Autodesk Inventor part; units mm, degrees
ref_plane "to_bolt_XY" through (5, -9, 0) normal (1, 0, 0) x (0, 0, -1)
ref_plane "to_bolt_YZ" through (5, -9, 0) normal (0, 0, -1) x (0, 1, 0)
ref_plane "to_bolt_ZX" through (5, -9, 0) normal (0, 1, 0) x (1, 0, 0)
sketch "Sketch_14" plane through (0, 0, 0) normal (1, 0, 0) x (0, 1, 0)
  line L0 (0, -4) -> (0, 4)
  line L1 (0, 4) -> (14.5, 4)
  line L2 (14.5, 4) -> (15, 3.5)
  line L3 (15, 3.5) -> (15, -3.5)
  line L4 (15, -3.5) -> (14.5, -4)
  line L5 (14.5, -4) -> (0, -4)
  line L6 (0, -4) -> (0, 4)
revolve "Revolution1" add sketch "Sketch_14" angle 360 about axis through (0, 0, -4) along (0, 0, -1)
sketch "Sketch_15" plane through (0, 0, 0) normal (1, 0, 0) x (0, 1, 0)
  line L0 (0, -4) -> (0, 4)
  line L1 (0, 4) -> (5.5, 4)
  line L2 (5.5, 4) -> (5, 3.5)
  line L3 (5, 3.5) -> (5, -3.5)
  line L4 (5, -3.5) -> (5.5, -4)
  line L5 (5.5, -4) -> (0, -4)
  line L6 (0, -4) -> (0, 4)
revolve "Revolution2" cut sketch "Sketch_15" angle 360 about axis through (0, 0, -4) along (0, 0, -1)
sketch "Sketch_16" plane through (0, 0, 0) normal (0, 0, 1) x (1, 0, 0)
  arc A0 (-0.75, -15.9824) -> (0.75, -15.9824) centre (0, 0) ccw
  line L0 (0.75, -15.9824) -> (0.75, 0)
  line L1 (0.75, 0) -> (-0.75, 0)
  line L2 (-0.75, 0) -> (-0.75, -15.9824)
extrude "Extrusion1" cut sketch "Sketch_16" along normal mid plane 8
sketch "Sketch4" plane through (0, 0, -4) normal (0, 0, -1) x (-1, 0, 0)
  point P0 (-10, 0)
hole "Hole1" at (10, 0, -4) direction (0, 0, 1) diameter 5.5 depth 8
sketch "Sketch5" plane through (0, 0, -4) normal (0, 0, -1) x (-1, 0, 0)
  point P0 (10, 0)
hole "Hole2" at (-10, 0, -4) direction (0, 0, 1) diameter 5.5 depth 8
sketch "Sketch6" plane through (0, 0, -4) normal (0, 0, -1) x (-1, 0, 0)
  point P0 (0, 10)
hole "Hole3" at (0, 10, -4) direction (0, 0, 1) diameter 5.5 depth 8
sketch "Sketch_23" plane through (0, -9, 0) normal (0, 1, 0) x (1, 0, 0)
  line L0 (15, 0) -> (0, 0)
  line L1 (0, 0) -> (0, 1.7)
  line L2 (0, 1.7) -> (5, 1.7)
  line L3 (5, 1.7) -> (5, 3)
  line L4 (5, 3) -> (15, 3)
  line L5 (15, 3) -> (15, 0)
  line L6 (15, 0) -> (0, 0)
revolve "Revolution3" cut sketch "Sketch_23" angle 360 about axis through (15, -9, 0) along (1, 0, 0)
sketch "Sketch8" plane through (-0.75, -14.4806, 4) normal (1, 0, 0) x (0, 0, -1)
  point P0 (4, 5.4806)
hole "Hole4" at (-0.75, -9, 0) direction (-1, 0, 0) diameter 2.459 depth 12.2404 countersink diameter 3 countersink angle 90
ref_plane "to_bolt_XY" through (5, -9, 0) normal (1, 0, 0) x (0, 0, -1)
ref_plane "to_bolt_YZ" through (5, -9, 0) normal (0, 0, -1) x (0, 1, 0)
ref_plane "to_bolt_ZX" through (5, -9, 0) normal (0, 1, 0) x (1, 0, 0)
properties part number "SCST10-8b"
Verification items for the finished model (mm, model axes). A direction names the side the tool comes from. Coordinates: 2 decimals unless noted, no trailing zeros. Write each loop counter-clockwise with the first axis right and the second up, starting at its lowest first coordinate (ties: lowest second). Pieces come first, ordered by that corner, then holes. Notation, with made-up numbers: (57.5, 66) -> (97.5, 66) arc R30 cw to (97.5, 100) -> close; hole circle Ø1 at (74.5, 81). An arc over 180 degrees is marked (long way). One line per item, written item: value. Start each with the question number.
Q1. Thickness scan on L1, parallel to X at y = 0, z = -0.25; L2, parallel to Z at x = -7.25, y = -9; L3, parallel to Y at x = -1, z = 1.5. Record the ranges inside material, lowest first. Write a range as from..to.
Q2. Cross-section at A-A on y = 0. Enter the section's corners in (x, z).
Q3. Access from +Z, -Z, +X, -X, +Y, -Y to the whole of each face (thin tool, end or side, straight path). Record for faces 1 (the cylindrical face through (2.9, -10.66, 0.37)), 2 (the cylindrical face through (0, 5, 0)), 3 (the flat face through (0.75, -11, 0)).
Q4. Mould release check, pull along X, two halves, no side actions. Record for faces 4 (the flat face through (5, -11, 0)), 5 (the conical face through (-0.634, 14.629, 3.858)), 6 (the flat face through (-0.75, -11, 0)): pulls with the +X half, pulls with the -X half, needs draft (parallel to the pull), parting line crosses it, or undercut.
Q5. Go/stop test with flat-tipped pins: P1, Ø2, axis at y = -4, z = -2.5, coming from the +X side; P2, Ø1, axis at y = 7, z = 0, coming from the -X side; P3, Ø4.5, axis at y = -9, z = 0, coming from the +X side. Record where each tip stops, or that it passes through.
Q6. Cross-section at B-B on x = -3.5. State how many separate pieces and enclosed holes the cut face has, and give its area (3 significant figures).
Checked values:
1. L1: x = -15..-12.75, -7.25..-5, 5..7.25, 12.75..15
1. L2: z = -4..-1.23, 1.23..4
1. L3: y = -14.97..-4.9, 4.9..7.44, 12.56..14.97
2. outline: (-15, -3.5) -> (-14.5, -4) -> (-12.75, -4) -> (-12.75, 4) -> (-14.5, 4) -> (-15, 3.5) -> close; (-7.25, -4) -> (-5.5, -4) -> (-5, -3.5) -> (-5, 3.5) -> (-5.5, 4) -> (-7.25, 4) -> close; (5, -3.5) -> (5.5, -4) -> (7.25, -4) -> (7.25, 4) -> (5.5, 4) -> (5, 3.5) -> close; (12.75, -4) -> (14.5, -4) -> (15, -3.5) -> (15, 3.5) -> (14.5, 4) -> (12.75, 4) -> close
3. face 1: +X
3. face 2: +Z, -Z
3. face 3: +Z, -Z, -Y
4. face 4: pulls with the +X half
4. face 5: parting line crosses it
4. face 6: undercut
5. P1: stops at x = 14.7
5. P2: stops at x = -13.52
5. P3: stops at x = 5
6. separate pieces: 2
6. enclosed holes: 1
6. area: 170 mm²
